Build history of the part. All positions in model axes, mm. A direction names the side the tool comes from. Round coordinates to 2 decimals unless told otherwise and drop trailing zeros. Loops run counter-clockwise (first coordinate to the right, second up) from the corner with the lowest first, then second, coordinate; pieces in that order, holes last.
from build123d import *

# Parameters (mm, degrees)
F0_R     = 1.6
F0_W     = 2.644199878
F0_H     = 1.5956377611
F1_DEPTH = 2
F2_R     = 2
F3_R     = 2


with BuildPart() as f1:
    # F0 (on Top) → F1 (new body)
    with BuildSketch(Plane.XY):
        with BuildLine():
            Line((10.0678037852, 41.4781346917), (10.0678037852, 40.3846651316))
            Line((10.0678037852, 40.3846651316), (10.0678037852, 35.5912074447))
            Line((10.0678037852, 35.5912074447), (19.349999167, 35.5912074447))
            ThreePointArc((19.349999167, 35.5912074447), (22.885533073, 34.1267413506), (24.349999167, 30.5912074447))
            Line((24.349999167, 30.5912074447), (24.349999167, 16.2233320251))
            ThreePointArc((24.349999167, 16.2233320251), (22.885533073, 12.6877981192), (19.349999167, 11.2233320251))
            Line((19.349999167, 11.2233320251), (10.0678037852, 11.2233320251))
            Line((10.0678037852, 11.2233320251), (10.0678037852, 5.7744667865))
            Line((10.0678037852, 5.7744667865), (46.6321945488, 5.7744667865))
            Line((46.6321945488, 5.7744667865), (46.6321945488, 11.2233320251))
            Line((46.6321945488, 11.2233320251), (37.349999167, 11.2233320251))
            ThreePointArc((37.349999167, 11.2233320251), (33.8144652611, 12.6877981192), (32.349999167, 16.2233320251))
            Line((32.349999167, 16.2233320251), (32.349999167, 24.7527061179))
            Line((32.349999167, 24.7527061179), (32.349999167, 30.5912074447))
            ThreePointArc((32.349999167, 30.5912074447), (33.8144652611, 34.1267413506), (37.349999167, 35.5912074447))
            Line((37.349999167, 35.5912074447), (46.6321945488, 35.5912074447))
            Line((46.6321945488, 35.5912074447), (46.6321945488, 40.3846651316))
            Line((46.6321945488, 40.3846651316), (46.6321945488, 41.4781346917))
            Line((46.6321945488, 41.4781346917), (38.1808124264, 41.4781346917))
            ThreePointArc((38.1808124264, 41.4781346917), (35.3876764753, 42.3310403404), (33.5474530963, 44.5987780681))
            ThreePointArc((33.5474530963, 44.5987780681), (32.3571350428, 48.4950101781), (31.87418136, 52.5402836502))
            Line((31.87418136, 52.5402836502), (28.349999167, 52.5402836502))
            Line((28.349999167, 52.5402836502), (24.825816974, 52.5402836502))
            ThreePointArc((24.825816974, 52.5402836502), (24.3428632913, 48.4950101781), (23.1525452378, 44.5987780681))
            ThreePointArc((23.1525452378, 44.5987780681), (21.3123218588, 42.3310403404), (18.5191859077, 41.4781346917))
            Line((18.5191859077, 41.4781346917), (10.0678037852, 41.4781346917))
        make_face()
        with Locations((13.099999167, 8.40333011)):
            Circle(F0_R, mode=Mode.SUBTRACT)
        with Locations((20.1146285981, 8.2314335741)):
            Rectangle(F0_W, F0_H, mode=Mode.SUBTRACT)
        with Locations((36.585369736, 8.2314335741)):
            Rectangle(F0_W, F0_H, mode=Mode.SUBTRACT)
        with Locations((43.599999167, 8.40333011)):
            Circle(F0_R, mode=Mode.SUBTRACT)
        with Locations((13.099999167, 38.90333011)):
            Circle(F0_R, mode=Mode.SUBTRACT)
        with BuildLine():
            add(Edge.make_bspline(
                [(26.9028567943, 41.4408115782), (27.8500015435, 41.4408115782), (27.8500015435, 40.7044507948)],
                knots=[0, 0, 0, 1, 1, 1], degree=2))
            add(Edge.make_bspline(
                [(27.8500015435, 40.7044507948), (27.8500015435, 40.3205030986), (27.5880429928, 40.1138684235)],
                knots=[0, 0, 0, 1, 1, 1], degree=2))
            add(Edge.make_bspline(
                [(27.5880429928, 40.1138684235), (27.3260844422, 39.9072337483), (26.8386810987, 39.9072337483)],
                knots=[0, 0, 0, 1, 1, 1], degree=2))
            Line((26.8386810987, 39.9072337483), (26.5410386483, 39.9072337483))
            Line((26.5410386483, 39.9072337483), (26.5410386483, 38.913063705))
            Line((26.5410386483, 38.913063705), (26.2472688693, 38.913063705))
            Line((26.2472688693, 38.913063705), (26.2472688693, 41.4408115782))
            Line((26.2472688693, 41.4408115782), (26.9028567943, 41.4408115782))
        make_face(mode=Mode.SUBTRACT)
        with Locations((28.349999167, 49.90333011)):
            Circle(F0_R, mode=Mode.SUBTRACT)
        with BuildLine():
            add(Edge.make_bspline(
                [(30.2671016656, 41.1348705465), (30.5730426973, 40.7890963244), (30.5730426973, 40.1805336935)],
                knots=[0, 0, 0, 1, 1, 1], degree=2))
            add(Edge.make_bspline(
                [(30.5730426973, 40.1805336935), (30.5730426973, 39.6947900663), (30.3777494167, 39.37308173)],
                knots=[0, 0, 0, 1, 1, 1], degree=2))
            add(Edge.make_bspline(
                [(30.3777494167, 39.37308173), (30.1824561361, 39.0513733938), (29.8261703776, 38.9374062102)],
                knots=[0, 0, 0, 1, 1, 1], degree=2))
            Line((29.8261703776, 38.9374062102), (30.4275409047, 38.3111399391))
            Line((30.4275409047, 38.3111399391), (30.0004405856, 38.3111399391))
            Line((30.0004405856, 38.3111399391), (29.5080580933, 38.8820823347))
            Line((29.5080580933, 38.8820823347), (29.4129010274, 38.8782096634))
            add(Edge.make_bspline(
                [(29.4129010274, 38.8782096634), (28.8546831232, 38.8782096634), (28.5512316659, 39.2198345948)],
                knots=[0, 0, 0, 1, 1, 1], degree=2))
            add(Edge.make_bspline(
                [(28.5512316659, 39.2198345948), (28.2477802086, 39.5614595262), (28.2477802086, 40.183853126)],
                knots=[0, 0, 0, 1, 1, 1], degree=2))
            add(Edge.make_bspline(
                [(28.2477802086, 40.183853126), (28.2477802086, 40.801267577), (28.552061524, 41.1409561728)],
                knots=[0, 0, 0, 1, 1, 1], degree=2))
            add(Edge.make_bspline(
                [(28.552061524, 41.1409561728), (28.8563428395, 41.4806447686), (29.4162204599, 41.4806447686)],
                knots=[0, 0, 0, 1, 1, 1], degree=2))
            add(Edge.make_bspline(
                [(29.4162204599, 41.4806447686), (29.9611606339, 41.4806447686), (30.2671016656, 41.1348705465)],
                knots=[0, 0, 0, 1, 1, 1], degree=2))
        make_face(mode=Mode.SUBTRACT)
        with Locations((43.599999167, 38.90333011)):
            Circle(F0_R, mode=Mode.SUBTRACT)
    extrude(amount=F1_DEPTH)

    # F2
    f2_edges = [f1.edges().sort_by_distance(p)[0] for p in [
        (46.632195, 5.774467, 1),
        (10.067804, 5.774467, 1),
        (10.067804, 35.591207, 1),
        (46.632195, 35.591207, 1),
    ]]
    fillet(f2_edges, radius=F2_R)

    # F3
    f3_edges = [f1.edges().sort_by_distance(p)[0] for p in [
        (10.067804, 41.478135, 1),
        (46.632195, 41.478135, 1),
        (46.632195, 11.223332, 1),
        (10.067804, 11.223332, 1),
        (24.825817, 52.540284, 1),
        (31.874181, 52.540284, 1),
    ]]
    fillet(f3_edges, radius=F3_R)


solid = f1.part
(1) Slice it at C-C on y = 27. List the corners of the cut face in (x, z).
Responses:
outline: (24.35, 0) - (32.35, 0) - (32.35, 2) - (24.35, 2) - close
(2) Slice it at A-A on x = 43.6. List the corners of the cut face in (y, z).
Responses:
outline: (5.77, 0) - (6.8, 0) - (6.8, 2) - (5.77, 2) - close; (10, 0) - (11.22, 0) - (11.22, 2) - (10, 2) - close; (35.59, 0) - (37.3, 0) - (37.3, 2) - (35.59, 2) - close; (40.5, 0) - (41.48, 0) - (41.48, 2) - (40.5, 2) - close
(3) Probe line 1 (Y direction, x = 43.6, z = 0.7); line 2 (Y direction, x = 39, z = 1.25); line 3 (X direction, y = 8, z = 0.25). List the from-to ranges inside material, lowest first.
Responses:
line 1: y = 5.77 to 6.8, 10 to 11.22, 35.59 to 37.3, 40.5 to 41.48
line 2: y = 5.77 to 11.22, 35.59 to 41.48
line 3: x = 10.07 to 11.55, 14.65 to 18.79, 21.44 to 35.26, 37.91 to 42.05, 45.15 to 46.63
(4) Slice it at D-D on z = 1.4. Count the separate pieces of the cut face and the enclosed holes in it, plus the area to 3 significant figures.
Responses:
separate pieces: 1
enclosed holes: 9
area: 672 mm2
(5) Which spindle directions (+Z, -Z, +X, -X, +Y, -Y) get a long thin tool onto all of the face, cutting with end or side? Do faces 5 (the face through (28, 26, 2)), 6 (the face through (33.78, 34.09, 0.99)), 7 (the face through (35.42, 42.31, 0.99)), 8 (the face through (22.9, 12.7, 1)), 9 (the face through (21.437, 8, 1)). Say none if no direction does.
Responses:
face 5: +Z, +X, -X, +Y, -Y
face 6: +Z, -Z, +X
face 7: +Z, -Z, +X, +Y
face 8: +Z, -Z, -X
face 9: +Z, -Z
(6) Pin check, flat tips, straight feed: P1, Ø0.6, axis at y = 22.5, z = 1.5, coming from the -X side; P2, Ø0.6, axis at x = 15.5, z = 1, coming from the +Y side; P3, Ø3, axis at x = 13.1, y = 38.9, coming from the +Z side; P4, Ø1, axis at x = 20, z = 0.5, coming from the +Y side. Stop position of each tip, or through.
Responses:
P1: stops at x = 24.35
P2: stops at y = 41.48
P3: passes through
P4: stops at y = 41.89
(7) Slice it at B-B on x = 18. List the corners of the cut face in (y, z), plus the area to 3 significant figures.
Responses:
outline: (5.77, 0) - (11.22, 0) - (11.22, 2) - (5.77, 2) - close; (35.59, 0) - (41.48, 0) - (41.48, 2) - (35.59, 2) - close
area: 22.7 mm2
(8) Pull direction Y, two halves, no side cores. Call faces 1 (the face through (10.638, 6.376, 1.014)), 2 (the face through (10.64, 36.19, 1.01)), 3 (the face through (28, 26, 0)), 4 (the face through (31.33, 52.04, 1.01)): +Y half, -Y half, draft (parallel to the pull), parting line (faces both ways), or undercut.
Responses:
face 1: -Y half
face 2: undercut
face 3: draft
face 4: +Y half
